```python
from build123d import *

# Parameters (mm, degrees)
SKETCH2_W          = 10.25
SKETCH2_H          = 6.35
BOTTOMSHAFT_DEPTH  = 25.4
TOPSHAFT_DEPTH     = 35
CUT_EXTRUDE1_DEPTH = 69.305837964
MOUNTHOLE_REACH    = 60.259
MOUNTHOLE_BORE_R   = 1.25
MOUNTHOLES_COUNT   = 3
FILLET1_R          = 0.254
FILLET2_R          = 2.5


with BuildPart() as part:
    # Sketch2 → Collar (revolve)
    with BuildSketch(Plane(origin=(0, 0, 0), x_dir=(1, 0, 0), z_dir=(0, 1, 0)), mode=Mode.PRIVATE) as collar_sk:
        with Locations((5.125, 3.175)):
            Rectangle(SKETCH2_W, SKETCH2_H)
    revolve(collar_sk.sketch.rotate(Axis((0, 0, -6.35), (0, 0, 1)), 180), axis=Axis((0, 0, -6.35), (0, 0, 1)))

    # Sketch3 → BottomShaft (add)
    with BuildSketch(Plane(origin=(0, 0, -6.35), x_dir=(-1, 0, 0), z_dir=(0, 0, -1))):
        Polygon((-6.375, -3.680607966), (0, -7.361215932), (6.375, -3.680607966), (6.375, 3.680607966), (0, 7.361215932), (-6.375, 3.680607966), align=None)
    extrude(amount=BOTTOMSHAFT_DEPTH)

    # Sketch4 → TopShaft (add)
    with BuildSketch(Plane.XY):
        Polygon((0, -7.361215932), (6.375, -3.680607966), (6.375, 3.680607966), (0, 7.361215932), (-6.375, 3.680607966), (-6.375, -3.680607966), align=None)
    extrude(amount=TOPSHAFT_DEPTH)

    # Sketch5 → Cut-Extrude1 (cut, through all)
    with BuildSketch(Plane.XY.offset(35)):
        Polygon((-4.875, -2.814582562), (0, -5.629165125), (4.875, -2.814582562), (4.875, 2.814582562), (0, 5.629165125), (-4.875, 2.814582562), align=None)
    extrude(amount=-CUT_EXTRUDE1_DEPTH, mode=Mode.SUBTRACT)

    # MountHole bore (on position points) → MountHole (cut, up to next)
    with BuildSketch(Plane(origin=(-3.1875, 5.520911949, 22.7), x_dir=(0.866025403784, 0.5, 0), z_dir=(-0.5, 0.866025403784, 0)), mode=Mode.PRIVATE) as mounthole_sk1:
        Circle(MOUNTHOLE_BORE_R)
    mounthole_tool1 = extrude(mounthole_sk1.sketch, amount=-MOUNTHOLE_REACH, mode=Mode.PRIVATE) & part.part
    mounthole = mounthole_tool1.solids().sort_by_distance((-3.1875, 5.520912, 22.7))[0]
    add(mounthole, mode=Mode.SUBTRACT)

    # MountHoleS: MountHole ×3 about axis
    mountholes_axis = Axis((0, 0, -6.35), (0, 0, -1))
    for i in range(1, MOUNTHOLES_COUNT):
        add(mounthole.rotate(mountholes_axis, i * 360 / MOUNTHOLES_COUNT), mode=Mode.SUBTRACT)

    # Fillet1
    fillet1_edges = [part.edges().sort_by_distance(p)[0] for p in [
        (6.375, 0, -31.75),
        (3.1875, -5.520911949, -31.75),
        (-3.1875, -5.520911949, -31.75),
        (-6.375, 0, -31.75),
        (-3.1875, 5.520911949, -31.75),
        (3.1875, 5.520911949, -31.75),
        (-3.1875, -5.520911949, 35),
        (3.1875, -5.520911949, 35),
        (6.375, 0, 35),
        (3.1875, 5.520911949, 35),
        (-3.1875, 5.520911949, 35),
        (-6.375, 0, 35),
        (10.25, 0, 0),
        (10.25, 0, -6.35),
        (-2.4375, -4.221873843, -31.75),
        (-4.875, 0, -31.75),
        (-2.4375, 4.221873843, -31.75),
        (2.4375, 4.221873843, -31.75),
        (4.875, 0, -31.75),
        (2.4375, -4.221873843, -31.75),
        (-2.4375, -4.221873843, 35),
        (2.4375, -4.221873843, 35),
        (4.875, 0, 35),
        (2.4375, 4.221873843, 35),
        (-2.4375, 4.221873843, 35),
        (-4.875, 0, 35),
    ]]
    fillet(fillet1_edges, radius=FILLET1_R)

    # Fillet2
    # the kernel refuses this fillet: 2.5 mm, written as the material it takes off along each edge
    with BuildSketch(Plane(origin=(-3.875, -2.237232293, -31.75), x_dir=(-0.5000000000000004, -0.8660254037844384, 0), z_dir=(0.8660254037844384, -0.5000000000000004, 0))) as fillet2_piece_1:
        with BuildLine():
            CenterArc((2.246, -0.254), 0.254, 0, 90)
            Line((2.5, -0.254), (2.5, 0))
            Line((2.5, 0), (2.246, 0))
        make_face()
    revolve(axis=Axis((-3.875, -2.237232293, -31.75), (0, 0, -1)), revolution_arc=60, mode=Mode.SUBTRACT)
    with BuildSketch(Plane(origin=(0, -4.474464586, -31.75), x_dir=(0.5000000000000002, -0.8660254037844386, 0), z_dir=(0.8660254037844386, 0.5000000000000002, 0))) as fillet2_piece_2:
        with BuildLine():
            CenterArc((2.246, -0.254), 0.254, 0, 90)
            Line((2.5, -0.254), (2.5, 0))
            Line((2.5, 0), (2.246, 0))
        make_face()
    revolve(axis=Axis((0, -4.474464586, -31.75), (0, 0, -1)), revolution_arc=60, mode=Mode.SUBTRACT)
    with BuildSketch(Plane(origin=(-3.875, 2.237232293, -31.75), x_dir=(-1, 0, 0), z_dir=(0, -1, 0))) as fillet2_piece_3:
        with BuildLine():
            CenterArc((2.246, -0.254), 0.254, 0, 90)
            Line((2.5, -0.254), (2.5, 0))
            Line((2.5, 0), (2.246, 0))
        make_face()
    revolve(axis=Axis((-3.875, 2.237232293, -31.75), (0, 0, -1)), revolution_arc=60, mode=Mode.SUBTRACT)
    with BuildSketch(Plane(origin=(3.875, -2.237232293, -31.75), x_dir=(1, 0, 0), z_dir=(0, 1, 0))) as fillet2_piece_4:
        with BuildLine():
            CenterArc((2.246, -0.254), 0.254, 0, 90)
            Line((2.5, -0.254), (2.5, 0))
            Line((2.5, 0), (2.246, 0))
        make_face()
    revolve(axis=Axis((3.875, -2.237232293, -31.75), (0, 0, -1)), revolution_arc=60, mode=Mode.SUBTRACT)
    with BuildSketch(Plane(origin=(0, 4.474464586, -31.75), x_dir=(-0.5, 0.8660254037844387, 0), z_dir=(-0.8660254037844387, -0.5, 0))) as fillet2_piece_5:
        with BuildLine():
            CenterArc((2.246, -0.254), 0.254, 0, 90)
            Line((2.5, -0.254), (2.5, 0))
            Line((2.5, 0), (2.246, 0))
        make_face()
    revolve(axis=Axis((0, 4.474464586, -31.75), (0, 0, -1)), revolution_arc=60, mode=Mode.SUBTRACT)
    with BuildSketch(Plane(origin=(3.875, 2.237232293, -31.75), x_dir=(0.5000000000000001, 0.8660254037844386, 0), z_dir=(-0.8660254037844386, 0.5000000000000001, 0))) as fillet2_piece_6:
        with BuildLine():
            CenterArc((2.246, -0.254), 0.254, 0, 90)
            Line((2.5, -0.254), (2.5, 0))
            Line((2.5, 0), (2.246, 0))
        make_face()
    revolve(axis=Axis((3.875, 2.237232293, -31.75), (0, 0, -1)), revolution_arc=60, mode=Mode.SUBTRACT)
    with BuildSketch(Plane(origin=(3.875, 2.237232293, 35), x_dir=(1, 0, 0), z_dir=(0, -1, 0))) as fillet2_piece_7:
        with BuildLine():
            CenterArc((2.246, -0.254), 0.254, 0, 90)
            Line((2.5, -0.254), (2.5, 0))
            Line((2.5, 0), (2.246, 0))
        make_face()
    revolve(axis=Axis((3.875, 2.237232293, 35), (0, 0, 1)), revolution_arc=60, mode=Mode.SUBTRACT)
    with BuildSketch(Plane(origin=(3.875, -2.237232293, 35), x_dir=(0.4999999999999999, -0.8660254037844387, 0), z_dir=(-0.8660254037844387, -0.4999999999999999, 0))) as fillet2_piece_8:
        with BuildLine():
            CenterArc((2.246, -0.254), 0.254, 0, 90)
            Line((2.5, -0.254), (2.5, 0))
            Line((2.5, 0), (2.246, 0))
        make_face()
    revolve(axis=Axis((3.875, -2.237232293, 35), (0, 0, 1)), revolution_arc=60, mode=Mode.SUBTRACT)
    with BuildSketch(Plane(origin=(0, 4.474464586, 35), x_dir=(0.49999999999999994, 0.8660254037844389, 0), z_dir=(0.8660254037844389, -0.49999999999999994, 0))) as fillet2_piece_9:
        with BuildLine():
            CenterArc((2.246, -0.254), 0.254, 0, 90)
            Line((2.5, -0.254), (2.5, 0))
            Line((2.5, 0), (2.246, 0))
        make_face()
    revolve(axis=Axis((0, 4.474464586, 35), (0, 0, 1)), revolution_arc=60, mode=Mode.SUBTRACT)
    with BuildSketch(Plane(origin=(0, -4.474464586, 35), x_dir=(-0.5000000000000001, -0.8660254037844387, 0), z_dir=(-0.8660254037844387, 0.5000000000000001, 0))) as fillet2_piece_10:
        with BuildLine():
            CenterArc((2.246, -0.254), 0.254, 0, 90)
            Line((2.5, -0.254), (2.5, 0))
            Line((2.5, 0), (2.246, 0))
        make_face()
    revolve(axis=Axis((0, -4.474464586, 35), (0, 0, 1)), revolution_arc=60, mode=Mode.SUBTRACT)
    with BuildSketch(Plane(origin=(-3.875, 2.237232293, 35), x_dir=(-0.5, 0.8660254037844387, 0), z_dir=(0.8660254037844387, 0.5, 0))) as fillet2_piece_11:
        with BuildLine():
            CenterArc((2.246, -0.254), 0.254, 0, 90)
            Line((2.5, -0.254), (2.5, 0))
            Line((2.5, 0), (2.246, 0))
        make_face()
    revolve(axis=Axis((-3.875, 2.237232293, 35), (0, 0, 1)), revolution_arc=60, mode=Mode.SUBTRACT)
    with BuildSketch(Plane(origin=(-3.875, -2.237232293, 35), x_dir=(-1, 0, 0), z_dir=(0, 1, 0))) as fillet2_piece_12:
        with BuildLine():
            CenterArc((2.246, -0.254), 0.254, 0, 90)
            Line((2.5, -0.254), (2.5, 0))
            Line((2.5, 0), (2.246, 0))
        make_face()
    revolve(axis=Axis((-3.875, -2.237232293, 35), (0, 0, 1)), revolution_arc=60, mode=Mode.SUBTRACT)
    with BuildSketch(Plane(origin=(-6.375, -3.680607966, 0), x_dir=(0, 1, 0), z_dir=(0, 0, 1)), Plane(origin=(-6.375, 3.680607966, 0), x_dir=(0.8660254037844388, 0.49999999999999956, 0), z_dir=(0, 0, 1)), Plane(origin=(0, 7.361215932, 0), x_dir=(0.8660254037844389, -0.4999999999999996, 0), z_dir=(0, 0, 1)), Plane(origin=(6.375, 3.680607966, 0), x_dir=(0, -1, 0), z_dir=(0, 0, 1)), Plane(origin=(6.375, -3.680607966, 0), x_dir=(-0.8660254037844388, -0.49999999999999956, 0), z_dir=(0, 0, 1))) as fillet2_piece_13:
        with BuildLine():
            CenterArc((FILLET2_R * 0.57735026919, -FILLET2_R), FILLET2_R, 90, 60)
            Line((-FILLET2_R * 0.288675134595, -FILLET2_R * 0.5), (0, 0))
            Line((0, 0), (FILLET2_R * 0.57735026919, 0))
        make_face()
    extrude(amount=35, mode=Mode.SUBTRACT)
    with BuildSketch(Plane(origin=(0, -7.361215932, 0), x_dir=(0.8660254037844388, 0.49999999999999983, 0), z_dir=(0, 0, 1))) as fillet2_piece_14:
        with BuildLine():
            CenterArc((FILLET2_R * 0.57735026919, FILLET2_R), FILLET2_R, 210, 60)
            Line((-FILLET2_R * 0.288675134595, FILLET2_R * 0.5), (0, 0))
            Line((0, 0), (FILLET2_R * 0.57735026919, 0))
        make_face()
    extrude(amount=35, mode=Mode.SUBTRACT)
    with BuildSketch(Plane(origin=(6.375, 3.680607966, -6.35), x_dir=(-0.8660254037844386, 0.5000000000000003, 0), z_dir=(0, 0, -1)), Plane(origin=(0, 7.361215932, -6.35), x_dir=(-0.8660254037844387, -0.49999999999999994, 0), z_dir=(0, 0, -1)), Plane(origin=(-6.375, 3.680607966, -6.35), x_dir=(0, -1, 0), z_dir=(0, 0, -1)), Plane(origin=(-6.375, -3.680607966, -6.35), x_dir=(0.8660254037844386, -0.5000000000000003, 0), z_dir=(0, 0, -1)), Plane(origin=(0, -7.361215932, -6.35), x_dir=(0.8660254037844386, 0.5, 0), z_dir=(0, 0, -1))) as fillet2_piece_15:
        with BuildLine():
            CenterArc((FILLET2_R * 0.57735026919, -FILLET2_R), FILLET2_R, 90, 60)
            Line((-FILLET2_R * 0.288675134595, -FILLET2_R * 0.5), (0, 0))
            Line((0, 0), (FILLET2_R * 0.57735026919, 0))
        make_face()
    extrude(amount=25.4, mode=Mode.SUBTRACT)
    with BuildSketch(Plane(origin=(6.375, -3.680607966, -6.35), x_dir=(-0.8660254037844385, -0.5000000000000003, 0), z_dir=(0, 0, -1))) as fillet2_piece_16:
        with BuildLine():
            CenterArc((FILLET2_R * 0.57735026919, FILLET2_R), FILLET2_R, 210, 60)
            Line((-FILLET2_R * 0.288675134595, FILLET2_R * 0.5), (0, 0))
            Line((0, 0), (FILLET2_R * 0.57735026919, 0))
        make_face()
    extrude(amount=25.4, mode=Mode.SUBTRACT)


solid = part.part
```
Could you check a few things on this model? Use its own coordinates, in mm. A direction names the side the tool comes from. Coordinates: 2 decimals unless noted, no trailing zeros. Order: outer loops, then holes, each group sorted by start corner. A loop starts at its lowest first (then second) coordinate and runs counter-clockwise, first axis right, second up. Notation, with made-up numbers: M -23,-14.75 L 9,-14.75 A19 ccw 9,15.25 Z; hole C 17.5,88.5 d8. An arc over 180 degrees is marked long. Use a Markdown table: item, result. Add a question column.
Q1. I want a section at C-C on z = -1. List the corners of the cut face in (x, y) for me (3 decimals), then the cut area to 3 significant figures.
Q2. I'm going to push flat-ended pins straight in: pin 1 (3 mm diameter, centred on y = 1, z = 6, fed in from -X) (3 decimals); pin 2 (6 mm diameter, centred on x = -5.5, z = -21.5, fed in from -Y); pin 3 (3 mm diameter, centred on y = -1, z = 17.5, fed in from +X) (3 decimals). Where does each tip first touch, or does it pass through?
Q3. If I drill on L1, parallel to Z at x = 5.3, y = 0; L2, parallel to X at y = 0, z = 19.5 (3 decimals); L3, parallel to Y at x = 0, z = 23, over which ranges is the centre line in solid material (lowest first)?
Q4. I want a section at A-A on z = -25.5. List the corners of the cut face in (x, y) for me (3 decimals).
Q5. We'd pull the mould along X, two halves only. Please class faces 5 (the flat face through (-3.21, 5.51, -18.75)), 6 (the cylindrical face through (3.124, -5.474, -31.674)), 7 (the flat face through (4.875, 0, 2)): pulls with the +X half, pulls with the -X half, needs draft (parallel to the pull), parting line crosses it, or undercut.
Q6. Which directions (+Z, -Z, +X, -X, +Y, -Y) give clear straight access to the entire face, cutting with the end or side of a thin tool? Please do faces 1 (the cylindrical face through (2.51, -4.27, 34.93)), 2 (the flat face through (-2.403, 4.242, 2.089)), 3 (the flat face through (3.16, 5.537, -18.747)), 4 (the flat face through (7, 0, -6.35)).
Q7. I want a section at B-B on z = 22.7. Give the number of separate pieces and of enclosed holes in the cut face, then the cut area to 3 significant figures.
Checked values:
| question | item | result |
|---|---|---|
| 1 | outline | C 0,0 d20.5; hole M -4.875,-2.815 L 0,-5.629 L 4.875,-2.815 L 4.875,2.815 L 0,5.629 L -4.875,2.815 Z |
| 1 | area | 248 mm² |
| 2 | pin 1 | x = -6.375 |
| 2 | pin 2 | y = -5.92 |
| 2 | pin 3 | x = 6.375 |
| 3 | L1 | -31.75 to 21.45, 23.95 to 35 |
| 3 | L2 | -6.375 to -4.875, 4.875 to 6.375 |
| 3 | L3 | -6.97 to -5.63, 5.63 to 6.97 |
| 4 | outline | M -6.375,-2.237 A2.5 ccw -5.125,-4.402 L -1.25,-6.64 A2.5 ccw 1.25,-6.64 L 5.125,-4.402 A2.5 ccw 6.375,-2.237 L 6.375,2.237 A2.5 ccw 5.125,4.402 L 1.25,6.64 A2.5 ccw -1.25,6.64 L -5.125,4.402 A2.5 ccw -6.375,2.237 Z; hole M -4.875,-2.815 L 0,-5.629 L 4.875,-2.815 L 4.875,2.815 L 0,5.629 L -4.875,2.815 Z |
| 5 | face 5 | pulls with the -X half |
| 5 | face 6 | pulls with the +X half |
| 5 | face 7 | undercut |
| 6 | face 1 | +Z |
| 6 | face 2 | +Z, -Z |
| 6 | face 3 | -Z, +X, +Y |
| 6 | face 4 | -Z |
| 7 | separate pieces | 3 |
| 7 | enclosed holes | 0 |
| 7 | area | 45.2 mm² |
